Work out the finished part from the listing and answer in its coordinate system (mm). Face numbers are marked on the shaded views. A direction names the side the tool comes from. Coordinates: 2 decimals unless noted, no trailing zeros. Order: outer loops, then holes, each group sorted by start corner. A loop starts at its lowest first (then second) coordinate and runs counter-clockwise, first axis right, second up. Notation, with made-up numbers: M 76.5,89 L 92.5,89 A25 ccw 92.5,112 Z; hole C 1,-3.5 d9. An arc over 180 degrees is marked long. Write item = value, one per line. Start each with the question number.
Q1. Find section B-B on z = 1.5. Give the vertices of the cut face in (x, y).
Q2. Each of these flat-tipped pins is pushed along its axis until it touches: P1, Ø3, axis at x = 3.5, z = -0.5, coming from the +Y side; P2, Ø0.7, axis at y = -0.5, z = 0, coming from the -X side; P3, Ø2.5, axis at x = 0.5, y = 0, coming from the +Z side. Where does it stop, or does it pass through?
Q3. A tool of negligible diameter and unlimited length cuts with its end or side. For the marked faces 1 and 2, from which of +Z, -Z, +X, -X, +Y, -Y can it reach the whole face along a straight path? Write none if from no direction.
Q4. Find section A-A on z = -0.75. Give the vertices of the cut face in (x, y).
Q5. Find section C-C on z = 3.5. Give the vertices of the cut face in (x, y), and give its area (3 significant figures).
Q6. Determine the mould class of the marked faces 3, 4, 5 and 6 for opening direction X: released by +X, released by -X, zero draft, split by the parting line, or undercut.
Q7. Straight lines are drawn through the part: line 1 along Y through (x, z) = (0, 7.5); line 2 along Z through (x, y) = (0.5, -3); line 3 along Z through (x, y) = (0.75, -1.5). For each, find the intervals that lie inside material, in ascending order.
```python
from build123d import *

# Parameters (mm, degrees)
SKETCH2_W          = 23.6
SKETCH2_H          = 23.6
CUT_EXTRUDE1_DEPTH = 1.5
CUT_EXTRUDE2_DEPTH = 5.7


with BuildPart() as part:
    # Sketch1 → Revolve1 (revolve)
    with BuildSketch(Plane(origin=(0, 0, 0), x_dir=(0, 0, -1), z_dir=(1, 0, 0)), mode=Mode.PRIVATE) as revolve1_sk:
        with BuildLine():
            Line((-14.4, 0), (-14.4, 3.4785))
            Line((-14.4, 3.4785), (-14.002165841, 5.734729636))
            ThreePointArc((-14.002165841, 5.734729636), (-13.933761812, 5.853208889), (-13.80520429, 5.9))
            Line((-13.80520429, 5.9), (-12.9, 5.9))
            Line((-12.9, 5.9), (-12.9, 4.2535))
            ThreePointArc((-12.9, 4.2535), (-12.790165043, 3.988334957), (-12.525, 3.8785))
            Line((-12.525, 3.8785), (-12, 3.8785))
            Line((-12, 3.8785), (-12, 4.513578644))
            Line((-12, 4.513578644), (-11.858578644, 4.655))
            Line((-11.858578644, 4.655), (-11.6, 4.655))
            Line((-11.6, 4.655), (-11.6, 4.858043913))
            Line((-11.6, 4.858043913), (-11, 4.9))
            Line((-11, 4.9), (-0.6, 4.9))
            Line((-0.6, 4.9), (-0.5, 4.8))
            Line((-0.5, 4.8), (-0.4, 4.9))
            Line((-0.4, 4.9), (0, 4.9))
            Line((0, 4.9), (0, 2.5))
            Line((0, 2.5), (2.5095, 2.5))
            Line((2.5095, 2.5), (3, 2.0095))
            Line((3, 2.0095), (3, 0))
            Line((3, 0), (-14.4, 0))
        make_face()
    revolve(revolve1_sk.sketch.rotate(Axis((0, 0, -3), (0, 0, 1)), 270), axis=Axis((0, 0, -3), (0, 0, 1)))

    # Sketch2 → Cut-Extrude1 (cut)
    with BuildSketch(Plane.XY.offset(14.4)):
        Rectangle(SKETCH2_W, SKETCH2_H)
        with BuildLine():
            Line((-4.9, 1), (-4.9, -1))
            ThreePointArc((-4.9, -1), (0, -5.9), (4.9, -1))
            Line((4.9, -1), (4.9, 1))
            ThreePointArc((4.9, 1), (0, 5.9), (-4.9, 1))
        make_face(mode=Mode.SUBTRACT)
    extrude(amount=-CUT_EXTRUDE1_DEPTH, mode=Mode.SUBTRACT)

    # Sketch3 → Cut-Extrude2 (cut)
    with BuildSketch(Plane.XY.offset(-3)):
        Polygon((-1.25, -0.721687836), (0, -1.443375673), (1.25, -0.721687836), (1.25, 0.721687836), (0, 1.443375673), (-1.25, 0.721687836), align=None)
    extrude(amount=CUT_EXTRUDE2_DEPTH, mode=Mode.SUBTRACT)

    # Sketch4 → Cut-Revolve1 (revolve, cut)
    with BuildSketch(Plane(origin=(0, 0, 0), x_dir=(0, 0, -1), z_dir=(1, 0, 0)), mode=Mode.PRIVATE) as cut_revolve1_sk:
        with BuildLine():
            Line((-14.4, 0), (-14.4, 3.4785))
            ThreePointArc((-14.4, 3.4785), (-14.312132034, 3.266367966), (-14.1, 3.1785))
            Line((-14.1, 3.1785), (-2.7, 3.1785))
            Line((-2.7, 3.1785), (-2.7, 0))
            Line((-2.7, 0), (-14.4, 0))
        make_face()
    revolve(cut_revolve1_sk.sketch.rotate(Axis((0, 0, 2.7), (0, 0, 1)), 270), axis=Axis((0, 0, 2.7), (0, 0, 1)), mode=Mode.SUBTRACT)


solid = part.part
```
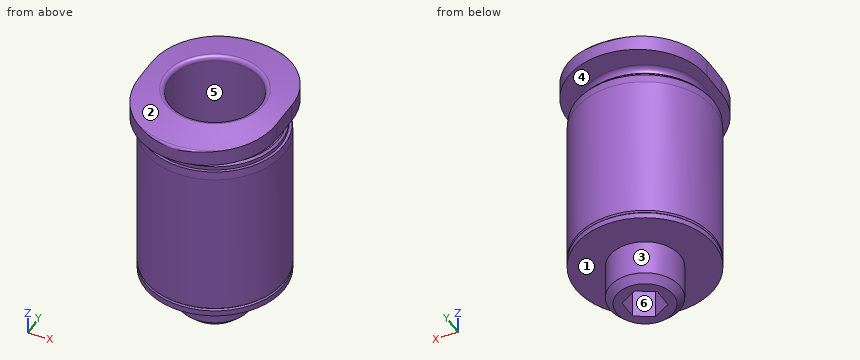
Findings below:
q1.outline = C 0,0 d9.8; hole M -1.25,-0.72 L 0,-1.44 L 1.25,-0.72 L 1.25,0.72 L 0,1.44 L -1.25,0.72 Z
q2.P1 = 4.43
q2.P2 = -4.9
q2.P3 = 2.7
q3.face_1 = -Z
q3.face_2 = +Z
q4.outline = C 0,0 d5; hole M -1.25,-0.72 L 0,-1.44 L 1.25,-0.72 L 1.25,0.72 L 0,1.44 L -1.25,0.72 Z
q5.outline = C 0,0 d9.8; hole C 0,0 d6.36
q5.area = 43.7 mm^2
q6.face_3 = split by the parting line
q6.face_4 = zero draft
q6.face_5 = undercut
q6.face_6 = undercut
q7.line_1 = -4.9 to -3.18, 3.18 to 4.9
q7.line_2 = 0 to 2.7
q7.line_3 = -3 to 2.7
